```python
from build123d import *

# Parameters (mm, degrees)
SKETCH1_R           = 2.254320316
BOSS_EXTRUDE1_DEPTH = 7.112
SKETCH2_R           = 0.268830558
SKETCH2_R_2         = 0.202182998
BOSS_EXTRUDE2_DEPTH = 10.16
FILLET4_R           = 1.778


with BuildPart() as part:
    # Sketch1 → Boss-Extrude1 (new body)
    with BuildSketch(Plane(origin=(0, 0, 0), x_dir=(1, 0, 0), z_dir=(0, 1, 0))):
        Circle(SKETCH1_R)
    extrude(amount=BOSS_EXTRUDE1_DEPTH)

    # Sketch2 → Boss-Extrude2 (add)
    with BuildSketch(Plane(origin=(0, 7.112, 0), x_dir=(1, 0, 0), z_dir=(0, 1, 0))):
        with Locations((0, 1.567947129)):
            Circle(SKETCH2_R)
        with Locations((0, -1.52494477)):
            Circle(SKETCH2_R_2)
    extrude(amount=BOSS_EXTRUDE2_DEPTH)

    # Fillet4
    fillet4_edges = [part.edges().sort_by_distance(p)[0] for p in [
        (-2.254320316, 0, 0),
    ]]
    fillet(fillet4_edges, radius=FILLET4_R)


solid = part.part
```
Source: CAD feature listing. Evaluate the final solid. Frame: model axes, mm. Round coordinates to 2 decimals unless told otherwise and drop trailing zeros. Write each loop counter-clockwise with the first axis right and the second up, starting at its lowest first coordinate (ties: lowest second). Pieces come first, ordered by that corner, then holes. Notation, with made-up numbers: M 12,53.5 L 24,53.5 A21 ccw 24,74.5 Z; hole C 78,19.5 d10. An arc over 180 degrees is marked long. Use CSV: the item, a comma, the result in double quotes. Start each with the question number.
Q1. Line query: line 1 (Z direction, x = 0.1, y = 7.5); line 2 (Y direction, x = -1.4, z = -0.25); line 3 (Y direction, x = 0.45, z = 0.2). Output: solid intervals per line, ascending. Write a range as from..to.
Q2. Cut plane A-A on y = 6. Output: boundary loops of the cut face in (x, z).
Q3. First-contact query: P1, Ø1, axis at x = -1, z = 0, coming from the +Y side. Flat tip, straight axial feed; report the tip coordinate or a pass-through.
Q4. Cut plane B-B on y = 10.25. Output: boundary loops of the cut face in (x, z), plus the area to 3 significant figures.
Results found:
1,line 1,"-1.82..-1.32, 1.35..1.7"
1,line 2,"0.27..7.11"
1,line 3,"0..7.11"
2,outline,"C 0,0 d4.51"
3,P1,"y = 7.11"
4,outline,"C 0,-1.57 d0.54; C 0,1.52 d0.4"
4,area,"0.355 mm^2"
